```python
from build123d import *

# Parameters (mm, degrees)
BOSS_EXTRUDE1_DEPTH   = 6
SKETCH2_W             = 12.8
SKETCH2_H             = 5.1
CUT_EXTRUDE1_DEPTH    = 142.370753694
F_1_CLEARANCE_HOLE1_D = 2
F_2_CLEARANCE_HOLE1_D = 2.4
F_1_CLEARANCE_HOLE2_D = 2.2
CHAMFER1_SIZE         = 0.4
CHAMFER2_SIZE         = 3
CHAMFER3_SIZE         = 2
FILLET1_R             = 3


with BuildPart() as part:
    # Sketch1 → Boss-Extrude1 (new body)
    with BuildSketch(Plane(origin=(0, 6, 0), x_dir=(1, 0, 0), z_dir=(0, 1, 0))):
        Polygon((16.9, -120), (0, -120), (0, -140), (18.7, -140), (18.7, -121.8), align=None)
    extrude(amount=-BOSS_EXTRUDE1_DEPTH)

    # Sketch2 → Cut-Extrude1 (cut, through all)
    with BuildSketch(Plane.XZ):
        with Locations((6.4, 122.55)):
            Rectangle(SKETCH2_W, SKETCH2_H)
    extrude(amount=-CUT_EXTRUDE1_DEPTH, mode=Mode.SUBTRACT)

    # #1 Clearance Hole1 (through all)
    with Locations(Plane(origin=(0, 6, 0), x_dir=(1, 0, 0), z_dir=(0, 1, 0))):
        with Locations((14.35, -138.5), (4.35, -138.5)):
            Hole(F_1_CLEARANCE_HOLE1_D / 2)

    # #2 Clearance Hole1 (through all)
    with Locations(Plane(origin=(0, 6, 0), x_dir=(1, 0, 0), z_dir=(0, 1, 0))):
        with Locations((3, -129)):
            Hole(F_2_CLEARANCE_HOLE1_D / 2)

    # #1 Clearance Hole2 (through all)
    with Locations(Plane(origin=(0, 6, 0), x_dir=(1, 0, 0), z_dir=(0, 1, 0))):
        with Locations((15.7, -123)):
            Hole(F_1_CLEARANCE_HOLE2_D / 2)

    # Chamfer1
    chamfer1_edges = [part.edges().sort_by_distance(p)[0] for p in [
        (6.4, 6, 125.1),
        (6.4, 0, 125.1),
    ]]
    chamfer(chamfer1_edges, length=CHAMFER1_SIZE)

    # Chamfer2
    chamfer2_edges = [part.edges().sort_by_distance(p)[0] for p in [
        (18.7, 3, 140),
    ]]
    chamfer(chamfer2_edges, length=CHAMFER2_SIZE)

    # Chamfer3
    chamfer3_edges = [part.edges().sort_by_distance(p)[0] for p in [
        (0, 3, 140),
    ]]
    chamfer(chamfer3_edges, length=CHAMFER3_SIZE)

    # Fillet1
    fillet1_edges = [part.edges().sort_by_distance(p)[0] for p in [
        (12.8, 3, 120),
    ]]
    fillet(fillet1_edges, radius=FILLET1_R)


solid = part.part
```
Geometry check sheet. Reference: the model listing, model coordinates, mm. A direction names the side the tool comes from. Give positions to 0.01 mm unless a question says otherwise; leave off trailing zeros. Loops run counter-clockwise (first coordinate to the right, second up) from the corner with the lowest first, then second, coordinate; pieces in that order, holes last. Notation, with made-up numbers: M 31,67 L 35,67 A19 ccw 35,87 Z; hole C 23,44 d3. An arc over 180 degrees is marked long. Answer as CSV lines item,"result".
Item 1: Access from +Z, -Z, +X, -X, +Y, -Y to the whole of each face (thin tool, end or side, straight path). Record for faces 1 (the cylindrical face through (3.26, 2.96, 130.17)), 2 (the flat face through (6, 3, 125.1)).
Values:
face 1,"+Y, -Y"
face 2,"-Z, -X, +Y, -Y"
Item 2: Depth check by flat-ended pin: P1, Ø2.5, axis at x = 4.35, z = 138.5, coming from the +Y side; P2, Ø2, axis at x = 3, z = 129, coming from the +Y side. Enter the tip coordinate at first touch or a pass-through.
Values:
P1,"stops at y = 6"
P2,"passes through"
Item 3: Release check for a two-part mould opening along X. For faces 3 (the cylindrical face through (14.567, 2.958, 139.476)), 4 (the flat face through (17.2, 3, 138.5)), 5 (the cylindrical face through (15.938, 2.958, 124.074)), 6 (the flat face through (9, 6, 132)) record: pulls with the +X half, pulls with the -X half, needs draft (parallel to the pull), parting line crosses it, or undercut.
Values:
face 3,"undercut"
face 4,"pulls with the +X half"
face 5,"undercut"
face 6,"needs draft"
Item 4: Cross-section at A-A on z = 138.5. Record the cut outline in (x, y), and give its area (3 significant figures).
Values:
outline,"M 0.5,0 L 3.35,0 L 3.35,6 L 0.5,6 Z; M 5.35,0 L 13.35,0 L 13.35,6 L 5.35,6 Z; M 15.35,0 L 17.2,0 L 17.2,6 L 15.35,6 Z"
area,"76.2 mm²"
Item 5: Material ranges on line 1 (X direction, y = 1.6, z = 129); line 2 (X direction, y = 2.7, z = 123); line 3 (Z direction, x = 4.35, y = 4.35), recorded low to high.
Values:
line 1,"x = 0 to 1.8, 4.2 to 18.7"
line 2,"x = 12.8 to 14.6, 16.8 to 18.7"
line 3,"z = 125.1 to 137.5, 139.5 to 140"
Item 6: Cross-section at D-D on z = 129. Record the cut outline in (x, y), and give its area (3 significant figures).
Values:
outline,"M 0,0 L 1.8,0 L 1.8,6 L 0,6 Z; M 4.2,0 L 18.7,0 L 18.7,6 L 4.2,6 Z"
area,"97.8 mm²"
Item 7: Cross-section at C-C on y = 4. Record the cut outline in (x, z).
Values:
outline,"M 0,125.1 L 12.8,125.1 L 12.8,123 A3 ccw 15.8,120 L 16.9,120 L 18.7,121.8 L 18.7,137 L 15.7,140 L 2,140 L 0,138 Z; hole C 3,129 d2.4; hole C 4.35,138.5 d2; hole C 14.35,138.5 d2; hole C 15.7,123 d2.2"
Item 8: Cross-section at B-B on x = 3. Record the cut outline in (y, z), and give its area (3 significant figures).
Values:
outline,"M 0,125.5 L 0.4,125.1 L 5.6,125.1 L 6,125.5 L 6,127.8 L 0,127.8 Z; M 0,130.2 L 6,130.2 L 6,140 L 0,140 Z"
area,"74.8 mm²"
